Geometry: final body of the model. Coordinates: model frame, mm. Face numbers are marked on the shaded views. A direction names the side the tool comes from. Give positions to 0.01 mm unless a question says otherwise; leave off trailing zeros. Order: outer loops, then holes, each group sorted by start corner. A loop starts at its lowest first (then second) coordinate and runs counter-clockwise, first axis right, second up. Notation, with made-up numbers: (-20.75, 70) - (36.25, 70) arc R15 ccw to (36.25, 94) - close; hole circle Ø4 at (-18, 52). An arc over 180 degrees is marked (long way). Put each result on its own line as item: value. Start each with the question number.
1. Section C-C on z = -29.25. Return the cut outline in (x, y).
2. Section D-D on x = 14.5. Return the cut outline in (y, z).
3. Section A-A on x = -47.75. Return the cut outline in (y, z).
4. First-contact query: P1, Ø4, axis at x = -25.5, z = 18, coming from the +Y side; P2, Ø5, axis at x = -8.25, z = 0, coming from the +Y side; P3, Ø2, axis at y = -3, z = 3.5, coming from the -X side; P4, Ø3.5, axis at y = -4, z = 0, coming from the +X side. Flat tips, straight axial feed; report the tip coordinate or a pass-through.
5. Ray query, line 1 along X through (y, z) = (-3.65, 29.25); line 2 along X through (y, z) = (-1.4, 0); line 3 along X through (y, z) = (-13.25, -11). Return the intervals inside material, ascending. Write a range as from..to.
6. Set-up query: the marked faces 1 and 2. Return all of +Z, -Z, +X, -X, +Y, -Y with unobstructed straight access to the full face (end or side cutting, diameter ignored); none if empty.
7. Section B-B on y = -7.5. Return the cut outline in (x, z).
8. Mould query, pull axis Z, two halves, no side actions, for the marked faces 3, 4, 5 and 6. Classes: pulls with the +Z half, pulls with the -Z half, needs draft (parallel to the pull), parting line crosses it, or undercut.
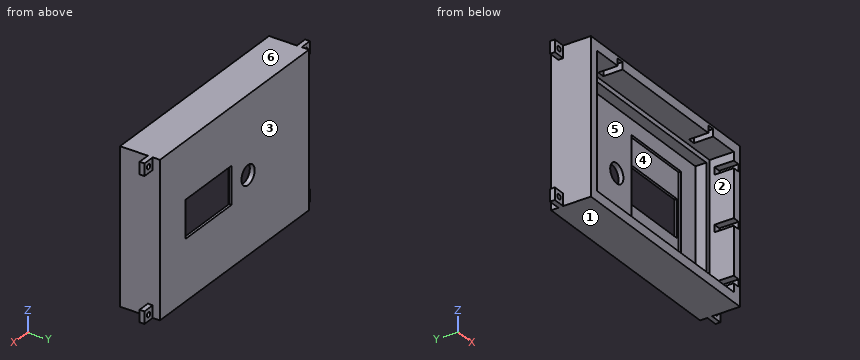
from build123d import *

# Parameters (mm, degrees)
SKETCH1_W           = 86.5
SKETCH1_H           = 59.5
BOSS_EXTRUDE3_DEPTH = 16.5
SKETCH5_W           = 83
SKETCH5_H           = 55.5
CUT_EXTRUDE2_DEPTH  = 10
SKETCH6_R           = 4
SKETCH6_W           = 28
SKETCH6_H           = 15.5
CUT_EXTRUDE5_DEPTH  = 6.5
SKETCH10_W          = 79
SKETCH10_H          = 52.175170105
CUT_EXTRUDE7_DEPTH  = 4.5
SKETCH12_W          = 30
SKETCH12_H          = 32.5
CUT_EXTRUDE9_DEPTH  = 1
SKETCH15_W          = 90.5
SKETCH15_H          = 63.5
SKETCH15_W_2        = 86.5
SKETCH15_H_2        = 59.5
BOSS_EXTRUDE4_DEPTH = 16.5
SKETCH16_W          = 3
SKETCH16_H          = 3
CUT_EXTRUDE11_DEPTH = 8
SKETCH21_W          = 5
SKETCH21_H          = 5
SKETCH21_R          = 1
BOSS_EXTRUDE6_DEPTH = 13.5
SKETCH23_W          = 5
SKETCH23_H          = 5
CUT_EXTRUDE12_DEPTH = 11.5
SKETCH24_W          = 5
SKETCH24_H          = 5
CUT_EXTRUDE13_DEPTH = 11.5
SKETCH25_W          = 5
SKETCH25_H          = 5
CUT_EXTRUDE14_DEPTH = 11.5
SKETCH26_W          = 5
SKETCH26_H          = 5
CUT_EXTRUDE15_DEPTH = 11.5


with BuildPart() as part:
    # Sketch1 → Boss-Extrude3 (new body)
    with BuildSketch(Plane(origin=(0, 0, 0), x_dir=(1, 0, 0), z_dir=(0, 1, 0))):
        Rectangle(SKETCH1_W, SKETCH1_H)
    extrude(amount=-BOSS_EXTRUDE3_DEPTH)

    # Sketch5 → Cut-Extrude2 (cut)
    with BuildSketch(Plane.XZ.offset(16.5)):
        Rectangle(SKETCH5_W, SKETCH5_H)
    extrude(amount=-CUT_EXTRUDE2_DEPTH, mode=Mode.SUBTRACT)

    # Sketch6 → Cut-Extrude5 (cut)
    with BuildSketch(Plane(origin=(0, 0, 0), x_dir=(1, 0, 0), z_dir=(0, 1, 0))):
        with Locations(Location((-8.25, 0, 0), (0, 0, 270))):
            Circle(SKETCH6_R)
        with Locations((15.75, -0.75)):
            Rectangle(SKETCH6_W, SKETCH6_H)
    extrude(amount=-CUT_EXTRUDE5_DEPTH, mode=Mode.SUBTRACT)

    # Sketch10 → Cut-Extrude7 (cut)
    with BuildSketch(Plane.XZ.offset(6.5)):
        with Locations((0, -0.337585053)):
            Rectangle(SKETCH10_W, SKETCH10_H)
    extrude(amount=-CUT_EXTRUDE7_DEPTH, mode=Mode.SUBTRACT)

    # Sketch12 → Cut-Extrude9 (cut)
    with BuildSketch(Plane.XZ.offset(2)):
        with Locations((15.75, 3.25)):
            Rectangle(SKETCH12_W, SKETCH12_H)
    extrude(amount=-CUT_EXTRUDE9_DEPTH, mode=Mode.SUBTRACT)

    # Sketch15 → Boss-Extrude4 (add)
    with BuildSketch(Plane.XZ.offset(16.5)):
        Rectangle(SKETCH15_W, SKETCH15_H)
        Rectangle(SKETCH15_W_2, SKETCH15_H_2, mode=Mode.SUBTRACT)
    extrude(amount=-BOSS_EXTRUDE4_DEPTH)

    # Sketch16 → Cut-Extrude11 (cut)
    with BuildSketch(Plane.XZ.offset(16.5)):
        with Locations((-27.5, 29.25)):
            Rectangle(SKETCH16_W, SKETCH16_H)
        with Locations((27.5, 29.25)):
            Rectangle(SKETCH16_W, SKETCH16_H)
        with Locations((43, 22.75)):
            Rectangle(SKETCH16_W, SKETCH16_H)
        with Locations((43, -22.75)):
            Rectangle(SKETCH16_W, SKETCH16_H)
        with Locations((43, 0)):
            Rectangle(SKETCH16_W, SKETCH16_H)
    extrude(amount=-CUT_EXTRUDE11_DEPTH, mode=Mode.SUBTRACT)

    # Sketch21 → Boss-Extrude6 (add)
    # profile 1 of 4: a face of its own
    with BuildSketch(Plane.XZ.offset(16.5)):
        with Locations((-47.75, 29.25)):
            Rectangle(SKETCH21_W, SKETCH21_H)
        with Locations(Location((-47.75, 29.25, 0), (0, 0, 270))):
            Circle(SKETCH21_R, mode=Mode.SUBTRACT)
    # profile 2 of 4: a face of its own
    with BuildSketch(Plane.XZ.offset(16.5)):
        with Locations((47.75, 29.25)):
            Rectangle(SKETCH21_W, SKETCH21_H)
        with Locations(Location((47.75, 29.25, 0), (0, 0, 90))):
            Circle(SKETCH21_R, mode=Mode.SUBTRACT)
    # profile 3 of 4: a face of its own
    with BuildSketch(Plane.XZ.offset(16.5)):
        with Locations((47.75, -29.25)):
            Rectangle(SKETCH21_W, SKETCH21_H)
        with Locations(Location((47.75, -29.25, 0), (0, 0, 270))):
            Circle(SKETCH21_R, mode=Mode.SUBTRACT)
    # profile 4 of 4: a face of its own
    with BuildSketch(Plane.XZ.offset(16.5)):
        with Locations((-47.75, -29.25)):
            Rectangle(SKETCH21_W, SKETCH21_H)
        with Locations(Location((-47.75, -29.25, 0), (0, 0, 90))):
            Circle(SKETCH21_R, mode=Mode.SUBTRACT)
    extrude(amount=-BOSS_EXTRUDE6_DEPTH)

    # Sketch23 → Cut-Extrude12 (cut)
    with BuildSketch(Plane(origin=(0, -16.5, 0), x_dir=(-1, 0, 0), z_dir=(0, -1, 0))):
        with Locations((-47.75, 29.25)):
            Rectangle(SKETCH23_W, SKETCH23_H)
    extrude(amount=-CUT_EXTRUDE12_DEPTH, mode=Mode.SUBTRACT)

    # Sketch24 → Cut-Extrude13 (cut)
    with BuildSketch(Plane.XZ.offset(16.5)):
        with Locations((47.75, 29.25)):
            Rectangle(SKETCH24_W, SKETCH24_H)
    extrude(amount=-CUT_EXTRUDE13_DEPTH, mode=Mode.SUBTRACT)

    # Sketch25 → Cut-Extrude14 (cut)
    with BuildSketch(Plane.XZ.offset(16.5)):
        with Locations((-47.75, 29.25)):
            Rectangle(SKETCH25_W, SKETCH25_H)
    extrude(amount=-CUT_EXTRUDE14_DEPTH, mode=Mode.SUBTRACT)

    # Sketch26 → Cut-Extrude15 (cut)
    with BuildSketch(Plane(origin=(0, -16.5, 0), x_dir=(-1, 0, 0), z_dir=(0, -1, 0))):
        with Locations((47.75, 29.25)):
            Rectangle(SKETCH26_W, SKETCH26_H)
    extrude(amount=-CUT_EXTRUDE15_DEPTH, mode=Mode.SUBTRACT)


solid = part.part
Resolved:
1. outline: (-50.25, -5) - (-48.75, -5) - (-48.75, -3) - (-50.25, -3) - close; (-46.75, -5) - (-45.25, -5) - (-45.25, -16.5) - (45.25, -16.5) - (45.25, -5) - (46.75, -5) - (46.75, -3) - (45.25, -3) - (45.25, 0) - (-45.25, 0) - (-45.25, -3) - (-46.75, -3) - close; (48.75, -5) - (50.25, -5) - (50.25, -3) - (48.75, -3) - close
2. outline: (-16.5, -31.75) - (0, -31.75) - (0, -7) - (-1, -7) - (-1, -13) - (-2, -13) - (-2, -26.43) - (-6.5, -26.43) - (-6.5, -27.75) - (-16.5, -27.75) - close; (-16.5, 27.75) - (-6.5, 27.75) - (-6.5, 25.75) - (-2, 25.75) - (-2, 19.5) - (-1, 19.5) - (-1, 8.5) - (0, 8.5) - (0, 31.75) - (-16.5, 31.75) - close
3. outline: (-5, -31.75) - (-3, -31.75) - (-3, -30.25) - (-5, -30.25) - close; (-5, -28.25) - (-3, -28.25) - (-3, -26.75) - (-5, -26.75) - close; (-5, 26.75) - (-3, 26.75) - (-3, 28.25) - (-5, 28.25) - close; (-5, 30.25) - (-3, 30.25) - (-3, 31.75) - (-5, 31.75) - close
4. P1: y = 0
4. P2: through
4. P3: x = -45.25
4. P4: x = 45.25
5. line 1: -50.25..-48.75, -46.75..46.75, 48.75..50.25
5. line 2: -45.25..-12.25, -4.25..0.75, 30.75..45.25
5. line 3: -45.25..-41.5, 41.5..45.25
6. face 1: -Z, +X, -X, +Y, -Y
6. face 2: -Y
7. outline: (-45.25, -31.75) - (45.25, -31.75) - (45.25, 31.75) - (-45.25, 31.75) - close; hole (-41.5, -27.75) - (41.5, -27.75) - (41.5, 27.75) - (-41.5, 27.75) - close
8. face 3: needs draft
8. face 4: undercut
8. face 5: undercut
8. face 6: pulls with the +Z half
